```python
from build123d import *

# Parameters (mm, degrees)
CROQUIS1_R              = 2.175
SALIENTE_EXTRUIR1_DEPTH = 2


with BuildPart() as part:
    # Croquis1 → Saliente-Extruir1 (new body)
    with BuildSketch(Plane(origin=(0, 0, 0), x_dir=(1, 0, 0), z_dir=(0, 1, 0))):
        with BuildLine():
            Line((0, 0), (0, 56))
            ThreePointArc((0, 56), (-2.928932188, 63.071067812), (-10, 66))
            Line((-10, 66), (-110, 66))
            ThreePointArc((-110, 66), (-117.071067812, 63.071067812), (-120, 56))
            Line((-120, 56), (-120, 10))
            ThreePointArc((-120, 10), (-117.071067812, 2.928932188), (-110, 0))
            Line((-110, 0), (-103.13836414, 0))
            Line((-103.13836414, 0), (-103.13836414, 24.315705481))
            Line((-103.13836414, 24.315705481), (-16.541911164, 24.315705481))
            Line((-16.541911164, 24.315705481), (-16.541911164, 0))
            Line((-16.541911164, 0), (0, 0))
        make_face()
        with Locations((-8.2, 8.2)):
            Circle(CROQUIS1_R, mode=Mode.SUBTRACT)
        with Locations((-8.2, 57.8)):
            Circle(CROQUIS1_R, mode=Mode.SUBTRACT)
        with Locations((-111.8, 57.8)):
            Circle(CROQUIS1_R, mode=Mode.SUBTRACT)
        with Locations((-111.8, 8.2)):
            Circle(CROQUIS1_R, mode=Mode.SUBTRACT)
    extrude(amount=SALIENTE_EXTRUIR1_DEPTH)


solid = part.part
```
Geometry: final body of the model. Coordinates: model frame, mm. Coordinates: 2 decimals unless noted, no trailing zeros. Order: outer loops, then holes, each group sorted by start corner. A loop starts at its lowest first (then second) coordinate and runs counter-clockwise, first axis right, second up.
Item 1: Section query C-C (z = -57.8). Output: boundary loops of the cut face in (x, y) (3 decimals), then the cut area to 3 significant figures.
Answer:
outline: (-119.837, 0) - (-113.975, 0) - (-113.975, 2) - (-119.837, 2) - close; (-109.625, 0) - (-10.375, 0) - (-10.375, 2) - (-109.625, 2) - close; (-6.025, 0) - (-0.163, 0) - (-0.163, 2) - (-6.025, 2) - close
area: 222 mm2
Item 2: Draft query along Z for faces 1 (the face through (-2.85, 0.99, -62.99)), 2 (the face through (-8.671, 0.986, -55.677)), 3 (the face through (-61, 0, -41)). Return one class per face: released by +Z, released by -Z, zero draft, split by the parting line, or undercut.
Answer:
face 1: released by -Z
face 2: undercut
face 3: zero draft
Item 3: Material intervals for line 1 along X through (y, z) = (0.75, -57.8) (3 decimals); line 2 along Z through (x, y) = (-8.2, 1.1) (3 decimals); line 3 along Z through (x, y) = (-53.5, 1.8), sorted ascending.
Answer:
line 1: x = -119.837 to -113.975, -109.625 to -10.375, -6.025 to -0.163
line 2: z = -65.837 to -59.975, -55.625 to -10.375, -6.025 to 0
line 3: z = -66 to -24.32
Item 4: Section query D-D (z = -8.2). Output: boundary loops of the cut face in (x, y) (3 decimals), then the cut area to 3 significant figures.
Answer:
outline: (-119.837, 0) - (-113.975, 0) - (-113.975, 2) - (-119.837, 2) - close; (-109.625, 0) - (-103.138, 0) - (-103.138, 2) - (-109.625, 2) - close; (-16.542, 0) - (-10.375, 0) - (-10.375, 2) - (-16.542, 2) - close; (-6.025, 0) - (0, 0) - (0, 2) - (-6.025, 2) - close
area: 49.1 mm2
Item 5: Section query B-B (x = -111.8). Output: boundary loops of the cut face in (y, z) (3 decimals), then the cut area to 3 significant figures.
Answer:
outline: (0, -65.837) - (2, -65.837) - (2, -59.975) - (0, -59.975) - close; (0, -55.625) - (2, -55.625) - (2, -10.375) - (0, -10.375) - close; (0, -6.025) - (2, -6.025) - (2, -0.163) - (0, -0.163) - close
area: 114 mm2
Item 6: Contact query for flat-ended pins moving along their axis: P1, Ø2.5, axis at x = -111.8, z = -8.2, coming from the +Y side; P2, Ø1, axis at x = -43.5, y = 0.5, coming from the +Z side; P3, Ø0.6, axis at y = 1, z = -6.5, coming from the -X side. Output: stop coordinate, or through.
Answer:
P1: passes through
P2: stops at z = -24.32
P3: stops at x = -119.47
Item 7: Section query A-A (y = 0.55). Output: boundary loops of the cut face in (x, z) (3 decimals), then the cut area to 3 significant figures.
Answer:
outline: (-120, -56) arc R10 ccw to (-110, -66) - (-10, -66) arc R10 ccw to (0, -56) - (0, 0) - (-16.542, 0) - (-16.542, -24.316) - (-103.138, -24.316) - (-103.138, 0) - (-110, 0) arc R10 ccw to (-120, -10) - close; hole circle Ø4.35 at (-111.8, -57.8); hole circle Ø4.35 at (-111.8, -8.2); hole circle Ø4.35 at (-8.2, -57.8); hole circle Ø4.35 at (-8.2, -8.2)
area: 5,690 mm2
